Could you check a few things on this model? Use its own coordinates, in mm. A direction names the side the tool comes from. Round coordinates to 2 decimals unless told otherwise and drop trailing zeros. Loops run counter-clockwise (first coordinate to the right, second up) from the corner with the lowest first, then second, coordinate; pieces in that order, holes last. Notation, with made-up numbers: (-18.75, -6) - (29.25, -6) arc R24 ccw to (29.25, 31) - close; hole circle Ø8 at (17, 67). An arc over 180 degrees is marked (long way). Use one line per item in the form item = value.
```python
from build123d import *

# Parameters (mm, degrees)
SKETCH_1_W          = 40
SKETCH_1_H          = 35
EXTRUDE_1_DEPTH     = 30
SKETCH_2_R          = 2.5
CUT_EXTRUDE_2_DEPTH = 20
SKETCH_3_R          = 5
CUT_EXTRUDE_3_DEPTH = 53.974050251


with BuildPart() as part:
    # 草图1 → 凸台-拉伸1 (new body)
    with BuildSketch(Plane.XY):
        Rectangle(SKETCH_1_W, SKETCH_1_H)
    extrude(amount=EXTRUDE_1_DEPTH)

    # 草图2 → 切除-拉伸2 (cut)
    with BuildSketch(Plane.XY):
        with Locations((-14, 10.5)):
            Circle(SKETCH_2_R)
        with Locations((14, 10.5)):
            Circle(SKETCH_2_R)
        with Locations((14, -10.5)):
            Circle(SKETCH_2_R)
        with Locations((-14, -10.5)):
            Circle(SKETCH_2_R)
    extrude(amount=CUT_EXTRUDE_2_DEPTH, mode=Mode.SUBTRACT)

    # 草图3 → 切除-拉伸3 (cut, through all)
    with BuildSketch(Plane(origin=(20, 0, 0), x_dir=(0, 0, -1), z_dir=(1, 0, 0))):
        with Locations((-15, 0)):
            Circle(SKETCH_3_R)
    extrude(amount=-CUT_EXTRUDE_3_DEPTH, mode=Mode.SUBTRACT)


solid = part.part
```
1. For P1, Ø9, axis at y = 0, z = 15, coming from the -X side; P2, Ø10, axis at x = 5.5, y = -11, coming from the -Z side; P3, Ø1.5, axis at x = -13.5, y = -11.5, coming from the -Z side, each with a flat end and sliding along its axis, tell me the tip position at first contact or that it passes through.
Solution:
P1 = through
P2 = 0
P3 = 20
2. If we section it at D-D, the plane z = 2: Write out the boundary of the cut face in (x, y).
Solution:
outline = (-20, -17.5) - (20, -17.5) - (20, 17.5) - (-20, 17.5) - close; hole circle Ø5 at (-14, -10.5); hole circle Ø5 at (-14, 10.5); hole circle Ø5 at (14, -10.5); hole circle Ø5 at (14, 10.5)
3. If we section it at B-B, the plane x = 14: Write out the boundary of the cut face in (y, z), plus the area to 3 significant figures.
Solution:
outline = (-17.5, 0) - (-13, 0) - (-13, 20) - (-8, 20) - (-8, 0) - (8, 0) - (8, 20) - (13, 20) - (13, 0) - (17.5, 0) - (17.5, 30) - (-17.5, 30) - close; hole circle Ø10 at (0, 15)
area = 771 mm^2
4. Please list where these lines run through material, in increasing order: line 1 along Y through (x, z) = (14, 8.25); line 2 along Y through (x, z) = (14, 13.5); line 3 along X through (y, z) = (-12.5, 9).
Solution:
line_1 = -17.5 to -13, -8 to 8, 13 to 17.5
line_2 = -17.5 to -13, -8 to -4.77, 4.77 to 8, 13 to 17.5
line_3 = -20 to -15.5, -12.5 to 12.5, 15.5 to 20
5. On a 3-axis mill with a long thin cutter (end or side, diameter ignored), from which of +Z, -Z, +X, -X, +Y, -Y can I reach the whole of each face in a straight line? I mean faces 1 (the face through (0, -17.5, 15)), 2 (the face through (-14, -10, 20)). Say none if no direction works.
Solution:
face_1 = +Z, -Z, +X, -X, -Y
face_2 = -Z
6. If we section it at A-A, the plane z = 15: Write out the boundary of the cut face in (x, y).
Solution:
outline = (-20, -17.5) - (20, -17.5) - (20, -5) - (-20, -5) - close; (-20, 5) - (20, 5) - (20, 17.5) - (-20, 17.5) - close; hole circle Ø5 at (-14, -10.5); hole circle Ø5 at (-14, 10.5); hole circle Ø5 at (14, -10.5); hole circle Ø5 at (14, 10.5)
7. If we section it at C-C, the plane y = 0: Write out the boundary of the cut face in (x, z), plus the area to 3 significant figures.
Solution:
outline = (-20, 0) - (20, 0) - (20, 10) - (-20, 10) - close; (-20, 20) - (20, 20) - (20, 30) - (-20, 30) - close
area = 800 mm^2
8. We'd pull the mould along X, two halves only. Please class faces 3 (the face through (-20, -4, 11)), 4 (the face through (0, 17.5, 15)), 5 (the face through (-14, 11, 20)), 6 (the face through (12, 9, 10)): +X half, -X half, draft (parallel to the pull), parting line (faces both ways), or undercut.
Solution:
face_3 = -X half
face_4 = draft
face_5 = undercut
face_6 = undercut
